from build123d import *

# Parameters (mm, degrees)
SKETCH_1_W          = 100
SKETCH_1_H          = 50
EXTRUDE_1_DEPTH     = 10
SHELL_1_T           = -4
FILLET_1_R          = 4.5
SKETCH_2_W          = 71.05
SKETCH_2_H          = 22.55
CUT_EXTRUDE_1_DEPTH = 4.5
EXTRUDE_3_DEPTH     = 2
SKETCH_7_R          = 1.55
CUT_EXTRUDE_2_DEPTH = 4
SKETCH_8_R          = 0.75
EXTRUDE_5_DEPTH     = 5
EXTRUDE_6_DEPTH     = 2.5


with BuildPart() as part:
    # Sketch 1 → Extrude 1 (new body)
    with BuildSketch(Plane(origin=(0, 0, 0), x_dir=(1, 0, 0), z_dir=(0, 1, 0))):
        with Locations((50, -25)):
            Rectangle(SKETCH_1_W, SKETCH_1_H)
    extrude(amount=EXTRUDE_1_DEPTH)

    # Shell 1
    shell_1_openings = [part.faces().sort_by_distance(p)[0] for p in [
        (50, 10, 25),
    ]]
    offset(amount=SHELL_1_T, openings=shell_1_openings, kind=Kind.INTERSECTION)

    # Fillet 1
    fillet_1_edges = [part.edges().sort_by_distance(p)[0] for p in [
        (50, 0, 0),
        (100, 0, 25),
        (50, 0, 50),
        (0, 0, 25),
        (0, 5, 0),
        (100, 5, 0),
        (100, 5, 50),
        (0, 5, 50),
    ]]
    fillet(fillet_1_edges, radius=FILLET_1_R)

    # Sketch 2 → Cut-Extrude 1 (cut)
    with BuildSketch(Plane(origin=(0, 0, 0), x_dir=(-1, 0, 0), z_dir=(0, -1, 0))):
        with Locations((-50, -25)):
            Rectangle(SKETCH_2_W, SKETCH_2_H)
    extrude(amount=-CUT_EXTRUDE_1_DEPTH, mode=Mode.SUBTRACT)

    # Sketch 6 → Extrude 3 (add)
    with BuildSketch(Plane(origin=(0, 4, 0), x_dir=(1, 0, 0), z_dir=(0, 1, 0))):
        Polygon((14.475, -13.725), (14.475, -14.725), (9.975, -14.725), (9.975, -6.725), (17.975, -6.725), (17.975, -13.725), align=None)
        Polygon((14.475, -36.275), (14.475, -34.275), (9.975, -34.275), (9.975, -41.775), (17.975, -41.775), (17.975, -36.275), align=None)
        Polygon((90.025, -41.775), (82.025, -41.775), (82.025, -36.275), (85.525, -36.275), (85.525, -34.275), (90.025, -34.275), align=None)
        Polygon((82.025, -6.725), (82.025, -13.725), (85.525, -13.725), (85.525, -14.725), (90.025, -14.725), (90.025, -6.725), align=None)
    extrude(amount=EXTRUDE_3_DEPTH)

    # Sketch 7 → Cut-Extrude 2 (cut)
    with BuildSketch(Plane(origin=(0, 6, 0), x_dir=(1, 0, 0), z_dir=(0, 1, 0))):
        with Locations(Location((12.475, -9.225, 0), (0, 0, 270))):
            Circle(SKETCH_7_R)
        with Locations(Location((87.525, -9.225, 0), (0, 0, 90))):
            Circle(SKETCH_7_R)
        with Locations(Location((12.475, -39.275, 0), (0, 0, 270))):
            Circle(SKETCH_7_R)
        with Locations(Location((87.525, -39.275, 0), (0, 0, 90))):
            Circle(SKETCH_7_R)
    extrude(amount=-CUT_EXTRUDE_2_DEPTH, mode=Mode.SUBTRACT)

    # Sketch 8 → Extrude 5 (add)
    with BuildSketch(Plane(origin=(0, 10, 0), x_dir=(1, 0, 0), z_dir=(0, 1, 0))):
        with Locations((6, -48)):
            Circle(SKETCH_8_R)
        with Locations((6, -2)):
            Circle(SKETCH_8_R)
        with Locations((94, -2)):
            Circle(SKETCH_8_R)
        with BuildLine():
            ThreePointArc((94.75, -2), (94.530330086, -2.530330086), (94, -2.75))
            Line((94, -2.75), (97.25, -2.75))
            Line((97.25, -2.75), (97.25, -6))
            ThreePointArc((97.25, -6), (97.469669914, -5.469669914), (98, -5.25))
            Line((98, -5.25), (98, -2))
            Line((98, -2), (94.75, -2))
        make_face()
        with Locations((98, -6)):
            Circle(SKETCH_8_R)
        with Locations((98, -44)):
            Circle(SKETCH_8_R)
        with BuildLine():
            Line((97.25, -47.25), (94, -47.25))
            ThreePointArc((94, -47.25), (94.530330086, -47.469669914), (94.75, -48))
            Line((94.75, -48), (98, -48))
            Line((98, -48), (98, -44.75))
            ThreePointArc((98, -44.75), (97.469669914, -44.530330086), (97.25, -44))
            Line((97.25, -44), (97.25, -47.25))
        make_face()
        with Locations((94, -48)):
            Circle(SKETCH_8_R)
        with BuildLine():
            Line((6, -47.25), (2.75, -47.25))
            Line((2.75, -47.25), (2.75, -48))
            Line((2.75, -48), (5.25, -48))
            ThreePointArc((5.25, -48), (5.469669914, -47.469669914), (6, -47.25))
        make_face()
        with BuildLine():
            Line((5.25, -2), (2.75, -2))
            Line((2.75, -2), (2.75, -2.75))
            Line((2.75, -2.75), (6, -2.75))
            ThreePointArc((6, -2.75), (5.469669914, -2.530330086), (5.25, -2))
        make_face()
    extrude(amount=EXTRUDE_5_DEPTH)

    # Sketch 8_4 → Extrude 6 (add)
    with BuildSketch(Plane(origin=(0, 10, 0), x_dir=(1, 0, 0), z_dir=(0, 1, 0))):
        with BuildLine():
            ThreePointArc((6.75, -2), (6.530330086, -2.530330086), (6, -2.75))
            Line((6, -2.75), (94, -2.75))
            ThreePointArc((94, -2.75), (93.469669914, -2.530330086), (93.25, -2))
            Line((93.25, -2), (6.75, -2))
        make_face()
        with BuildLine():
            ThreePointArc((98, -6.75), (97.469669914, -6.530330086), (97.25, -6))
            Line((97.25, -6), (97.25, -44))
            ThreePointArc((97.25, -44), (97.469669914, -43.469669914), (98, -43.25))
            Line((98, -43.25), (98, -6.75))
        make_face()
        with BuildLine():
            Line((94, -47.25), (6, -47.25))
            ThreePointArc((6, -47.25), (6.530330086, -47.469669914), (6.75, -48))
            Line((6.75, -48), (93.25, -48))
            ThreePointArc((93.25, -48), (93.469669914, -47.469669914), (94, -47.25))
        make_face()
    extrude(amount=EXTRUDE_6_DEPTH)


solid = part.part
Could you check a few things on this model? Use its own coordinates, in mm. A direction names the side the tool comes from. Give positions to 0.01 mm unless a question says otherwise; leave off trailing zeros. Order: outer loops, then holes, each group sorted by start corner. A loop starts at its lowest first (then second) coordinate and runs counter-clockwise, first axis right, second up.
1. For faces 1 (the cylindrical face through (98.647, 7.288, 48.717)), 2 (the flat face through (9.975, 5, 11)), 3 (the flat face through (85.525, 2, 25)), 4 (the flat face through (51, 11, 2)), 5 (the flat face through (49, 11, 2.75)), which set-ups out of +Z, -Z, +X, -X, +Y, -Y let a thin tool reach every point of the face, with its end or its side?
2. Suppose I cut it at A-A (x = 25.5). List the corners of the cut face in (y, z) for me (3 decimals).
3. I need wall thicknesses on L1, parallel to X at y = 5, z = 7.5 (3 decimals); L2, parallel to Z at x = 54.5, y = 9.75; L3, parallel to X at y = 3.25, z = 39.5. Which ranges of each line are inside material? Lowest first, please.
4. Suppose I cut it at B-B (z = 25). List the corners of the cut face in (x, y) for me (3 decimals), plus the area to 3 significant figures.
5. We'd pull the mould along X, two halves only. Please class faces 6 (the cylindrical face through (1.283, 7.288, 48.647)), 7 (the flat face through (49, 7, 46)), 8 (the cylindrical face through (98.717, 1.353, 24.713)): pulls with the +X half, pulls with the -X half, needs draft (parallel to the pull), parting line crosses it, or undercut.
6. Will these pins go through, and if not, where does the flat tip stop? P1, Ø5, axis at x = 87.525, z = 9.225, coming from the +Y side; P2, Ø10, axis at x = 24.5, z = 12.5, coming from the +Y side; P3, Ø3, axis at x = 45.5, y = 1.5, coming from the +Z side.
7. Suppose I cut it at C-C (y = 9). List the corners of the cut face in (x, z) for me.
8. Suppose I cut it at D-D (x = 83.5). List the corners of the cut face in (y, z) for me (3 decimals), plus the area to 3 significant figures.
Solved:
1. face 1: +Z, +X, +Y, -Y
1. face 2: +Y
1. face 3: +Y, -Y
1. face 4: -Z, +Y
1. face 5: -X, +Y
2. outline: (0, 4.5) arc R4.5 ccw to (4.5, 0) - (10, 0) - (10, 2) - (12.5, 2) - (12.5, 2.75) - (10, 2.75) - (10, 4) - (4, 4) - (4, 13.725) - (0, 13.725) - close; (0, 36.275) - (4, 36.275) - (4, 46) - (10, 46) - (10, 47.25) - (12.5, 47.25) - (12.5, 48) - (10, 48) - (10, 50) - (4.5, 50) arc R4.5 ccw to (0, 45.5) - close
3. L1: x = 0 to 4, 9.975 to 17.975, 82.025 to 90.025, 96 to 100
3. L2: z = 0 to 4, 46 to 50
3. L3: x = 0.18 to 10.94, 14.01 to 85.99, 89.06 to 99.82
4. outline: (0, 4.5) arc R4.5 ccw to (4.5, 0) - (14.475, 0) - (14.475, 4) - (4, 4) - (4, 10) - (0, 10) - close; (85.525, 0) - (95.5, 0) arc R4.5 ccw to (100, 4.5) - (100, 10) - (98, 10) - (98, 12.5) - (97.25, 12.5) - (97.25, 10) - (96, 10) - (96, 4) - (85.525, 4) - close
4. area: 157 mm2
5. face 6: pulls with the -X half
5. face 7: undercut
5. face 8: pulls with the +X half
6. P1: stops at y = 6
6. P2: stops at y = 4
6. P3: stops at z = 49.74
7. outline: (0, 4.5) arc R4.5 ccw to (4.5, 0) - (95.5, 0) arc R4.5 ccw to (100, 4.5) - (100, 45.5) arc R4.5 ccw to (95.5, 50) - (4.5, 50) arc R4.5 ccw to (0, 45.5) - close; hole (4, 4) - (96, 4) - (96, 46) - (4, 46) - close
8. outline: (0, 4.5) arc R4.5 ccw to (4.5, 0) - (10, 0) - (10, 2) - (12.5, 2) - (12.5, 2.75) - (10, 2.75) - (10, 4) - (4, 4) - (4, 6.725) - (6, 6.725) - (6, 13.725) - (0, 13.725) - close; (0, 36.275) - (6, 36.275) - (6, 41.775) - (4, 41.775) - (4, 46) - (10, 46) - (10, 47.25) - (12.5, 47.25) - (12.5, 48) - (10, 48) - (10, 50) - (4.5, 50) arc R4.5 ccw to (0, 45.5) - close
8. area: 178 mm2
